Design review of the part built by this model. Coordinates are the model's own, in mm. Coordinates: 2 decimals unless noted, no trailing zeros. Order: outer loops, then holes, each group sorted by start corner. A loop starts at its lowest first (then second) coordinate and runs counter-clockwise, first axis right, second up. Notation, with made-up numbers: (8, -5) -> (23, -5) arc R23 cw to (23, 25) -> close; hole circle Ø1 at (81, 4.5). An arc over 180 degrees is marked (long way). Write item = value, one per line.
Autodesk Inventor part; units mm, degrees
ref_plane "YZ Plane" through (0, 0, 0) normal (1, 0, 0) x (0, 1, 0)
ref_plane "XZ Plane" through (0, 0, 0) normal (0, 1, 0) x (-1, 0, 0)
ref_plane "XY Plane" through (0, 0, 0) normal (0, 0, 1) x (1, 0, 0)
sketch "Sketch1" plane through (0, 0, 0) normal (0, 0, 1) x (1, 0, 0)
  line L0 (0, 0) -> (38.1, 0)
  line L1 (38.1, 0) -> (38.1, 19.05)
  line L2 (38.1, 19.05) -> (0, 19.05)
  line L3 (0, 19.05) -> (0, 0)
  circle A0 centre (19.05, 6.35) radius 4.7625
  point P0 (0, 9.525)
  point P1 (19.05, 19.05)
  dimension "d0" = 19.05
  dimension "d1" = 38.1
  dimension "d2" = 9.525
  dimension "d5" = 6.35
extrude "Extrusion1" add sketch "Sketch1" along normal blind 12.7
sketch "Sketch2" plane through (0, 19.05, 0) normal (0, 1, 0) x (1, 0, 0)
  line L0 (38.1, 0) -> (38.1, -12.7)
  line L1 (0, 0) -> (0, -12.7)
  circle A0 centre (6.35, -6.35) radius 3.175
  circle A1 centre (31.75, -6.35) radius 3.175
  point P0 (0, -6.35)
  dimension "d6" = 6.35
  dimension "d7" = 6.35
  dimension "d8" = 6.35
  dimension "d9" = 6.35
extrude "Extrusion2" cut sketch "Sketch2" against normal through all
equation "\"d7\" = d6"
properties part number "8 ball arch mount"
(1) We need section D-D (x = 6.35). Write out the cut boundary in (y, z) (3 decimals).
Report:
outline = (0, 0) -> (19.05, 0) -> (19.05, 3.175) -> (0, 3.175) -> close; (0, 9.525) -> (19.05, 9.525) -> (19.05, 12.7) -> (0, 12.7) -> close
(2) We need section B-B (x = 19.05). Write out the cut boundary in (y, z), and give its area (3 significant figures).
Report:
outline = (0, 0) -> (1.59, 0) -> (1.59, 12.7) -> (0, 12.7) -> close; (11.11, 0) -> (19.05, 0) -> (19.05, 12.7) -> (11.11, 12.7) -> close
area = 121 mm²
(3) Insertion check: pin 1 (2 mm diameter, centred on y = 3, z = 6.5, fed in from -X). The pin has a flat end and moves straight along its axis. Give the tip position at first contact, or say it passes through.
Report:
pin_1 = 0
(4) We need section A-A (z = 6.35). Give the number of separate pieces and of enclosed holes in the cut face, and give its area (3 significant figures).
Report:
separate_pieces = 3
enclosed_holes = 1
area = 413 mm²
(5) The part is to be moulded in two halves that separate along X. For faces 1 (the cylindrical face through (14.292, 6.141, 6.261)), 2 (the flat face through (19, 12, 0)), 3 (the flat face through (0, 10, 6)), say which applies: released by +X, released by -X, zero draft, split by the parting line, or undercut.
Report:
face_1 = undercut
face_2 = zero draft
face_3 = released by -X
(6) We need section C-C (y = 2.75). Write out the cut boundary in (x, z) (3 decimals).
Report:
outline = (0, 0) -> (15.932, 0) -> (15.932, 12.7) -> (0, 12.7) -> close; (22.168, 0) -> (38.1, 0) -> (38.1, 12.7) -> (22.168, 12.7) -> close; hole circle Ø6.35 at (6.35, 6.35); hole circle Ø6.35 at (31.75, 6.35)
(7) For L1, parallel to X at y = 11.5, z = 6.35 (3 decimals); L2, parallel to Y at x = 19.05, z = 4.75; L3, parallel to Z at x = 31.75, y = 7.25 (3 decimals), list the stretches that pass through material, from the lowest coordinate up.
Report:
L1 = 0 to 3.175, 9.525 to 28.575, 34.925 to 38.1
L2 = 0 to 1.59, 11.11 to 19.05
L3 = 0 to 3.175, 9.525 to 12.7
